Verification items for this drawing (mm, ordinates from the low corner). A direction names the side the tool comes from. Round coordinates to 2 decimals unless told otherwise and drop trailing zeros. Loops run counter-clockwise (first coordinate to the right, second up) from the corner with the lowest first, then second, coordinate; pieces in that order, holes last. Notation, with made-up numbers: M -39.75,-5 L -3.75,-5 A28 cw -3.75,26 Z; hole C 63,1.5 d6. An arc over 180 degrees is marked long. Answer as CSV lines item,"result".
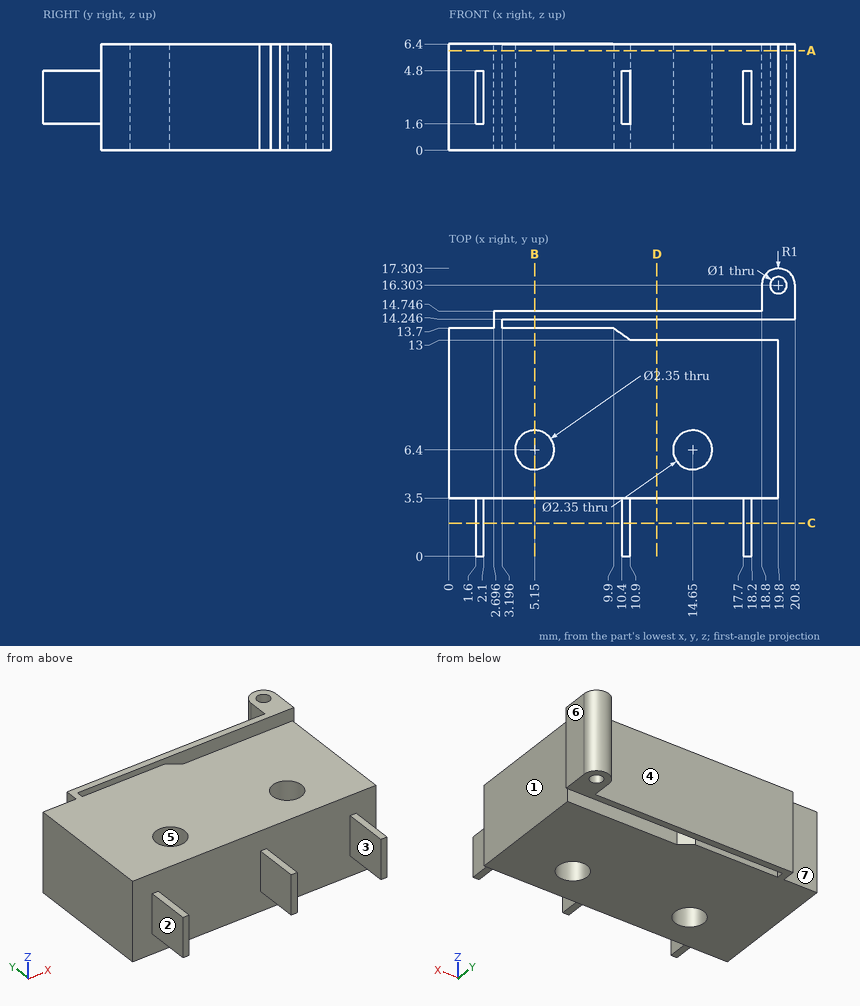
1) Section check C-C (y = 2). Record the cut outline in (x, z).
Here are the results:
outline,"M 1.6,1.6 L 2.1,1.6 L 2.1,4.8 L 1.6,4.8 Z; M 10.4,1.6 L 10.9,1.6 L 10.9,4.8 L 10.4,4.8 Z; M 17.7,1.6 L 18.2,1.6 L 18.2,4.8 L 17.7,4.8 Z"
2) Section check B-B (x = 5.15). Record the cut outline in (y, z) (1 decimal).
Here are the results:
outline,"M 3.5,0 L 5.2,0 L 5.2,6.4 L 3.5,6.4 Z; M 7.6,0 L 13.7,0 L 13.7,6.4 L 7.6,6.4 Z; M 14.2,0 L 14.7,0 L 14.7,6.4 L 14.2,6.4 Z"
3) Go/stop test with flat-tipped pins: pin 1 (1.7 mm diameter, centred on y = 15.5, z = 3.5, fed in from -X); pin 2 (3 mm diameter, centred on y = 11.5, z = 5, fed in from +X); pin 3 (3 mm diameter, centred on x = 13, z = 2, fed in from +Y). Record where each tip stops, or that it passes through.
Here are the results:
pin 1,"stops at x = 2.7"
pin 2,"stops at x = 19.8"
pin 3,"stops at y = 14.75"
4) Set-up check for the marked faces 1, 2, 3 and 4: record each of +Z, -Z, +X, -X, +Y, -Y from which the full face is reachable in a straight line by a thin tool's end or side.
Here are the results:
face 1,"+Z, -Z, +X, -Y"
face 2,"+Z, -Z, -X, -Y"
face 3,"+Z, -Z, -Y"
face 4,"+Z, -Z, -X, +Y"
5) Section check D-D (x = 12.5). Record the cut outline in (y, z).
Here are the results:
outline,"M 3.5,0 L 13,0 L 13,6.4 L 3.5,6.4 Z; M 14.25,0 L 14.75,0 L 14.75,6.4 L 14.25,6.4 Z"
6) Draft check along Y on the marked faces 5, 6 and 7. Enter one of: +Y half, -Y half, draft (parallel to the pull), parting line (faces both ways), or undercut.
Here are the results:
face 5,"undercut"
face 6,"draft"
face 7,"+Y half"
7) Section check A-A (z = 6). State how many separate pieces and enclosed holes the cut face has, plus the area to 3 significant figures.
Here are the results:
separate pieces,"1"
enclosed holes,"3"
area,"200 mm^2"
8) Material ranges on probe 1 along Y at (x, z) = (14.65, 2.75) (1 decimal); probe 2 along X at (y, z) = (1.5, 3); probe 3 along X at (y, z) = (7, 5), recorded low to high.
Here are the results:
probe 1,"y = 3.5 to 5.2, 7.6 to 13, 14.2 to 14.7"
probe 2,"x = 1.6 to 2.1, 10.4 to 10.9, 17.7 to 18.2"
probe 3,"x = 0 to 4.14, 6.16 to 13.64, 15.66 to 19.8"
